Model file for the job. Use its own axes, mm. A direction names the side the tool comes from. Round coordinates to 2 decimals unless told otherwise and drop trailing zeros. Order: outer loops, then holes, each group sorted by start corner. A loop starts at its lowest first (then second) coordinate and runs counter-clockwise, first axis right, second up. Notation, with made-up numbers: (76, 41) - (80, 41) arc R27 cw to (80, 67) - close; hole circle Ø11 at (30.25, 72.5). An arc over 180 degrees is marked (long way). Answer as CSV lines item,"result". Start each with the question number.
1. Pin check, flat tips, straight feed: pin 1 Ø8 at (x, z) = (-31.5, 25.5) entering from -Y; pin 2 Ø6.5 at (x, y) = (2.5, 23.5) entering from +Z; pin 3 Ø15.5 at (x, y) = (5.5, -18) entering from +Z. Stop position of each tip, or through.
2. Band-saw the part on B-B on z = 22.5. List the corners of the cut face in (x, y).
3. Pull direction Y, two halves, no side cores. Call faces 3 (the face through (24.84, 19.39, 47.26)), 4 (the face through (-10, 22, 48)), 5 (the face through (43.14, -9.58, 25.32)), 6 (the face through (-37, 24, 0)): released by +Y, released by -Y, zero draft, split by the parting line, or undercut.
4. Band-saw the part on A-A on y = 0. List the corners of the cut face in (x, z).
5. Wall check: line 1 along X through (y, z) = (0, 47.4); line 2 along Z through (x, y) = (15.5, -3.5); line 3 along X through (y, z) = (22.5, 48.5). Give the ranges that are in metal, low to high. Write a range as [from, to].
6. 3-axis set-ups, long thin cutter, end or side, ignore diameter. For faces 1 (the face through (-1, 1, 2)), 2 (the face through (7.91, 12.21, 48.74)): which of +Z, -Z, +X, -X, +Y, -Y reach the whole face in a straight line?
```python
from build123d import *

# Parameters (mm, degrees)
F3_DEPTH = 1.5
F5_DEPTH = 1.5


with BuildPart() as f1:
    # F0 (on Right) → F1 (revolve)
    with BuildSketch(Plane.YZ):
        Polygon((0, 48), (0, 2), (42.57288, 2), (43.38192, 0), (45, 0), (44.19096, 2), (44.19096, 48), (45, 50), (43.38192, 50), (42.57288, 48), align=None)
    revolve(axis=Axis((0, 0, 25), (0, 0, 1)))

    # F2 (on face) → F3 (cut)
    with BuildSketch(Plane.XY.offset(48)):
        with BuildLine():
            ThreePointArc((-22.449944, 20), (-24.806967, 19.409586), (-26.607341, 17.777778))
            ThreePointArc((-26.607341, 17.777778), (0, -32), (26.607341, 17.777778))
            ThreePointArc((26.607341, 17.777778), (24.806967, 19.409586), (22.449944, 20))
            Line((22.449944, 20), (-22.449944, 20))
        make_face()
    extrude(amount=-F3_DEPTH, mode=Mode.SUBTRACT)

    # F4 (on face) → F5 (join)
    with BuildSketch(Plane.XY.offset(48)):
        with BuildLine():
            Line((1.90098, 39), (-1.90098, 39))
            ThreePointArc((-1.90098, 39), (-5.070925, 37.866711), (-6.803884, 34.980581))
            Line((-6.803884, 34.980581), (-9.846991, 19.765045))
            ThreePointArc((-9.846991, 19.765045), (-7.981844, 12.2941), (-1.021765, 9))
            Line((-1.021765, 9), (1.021765, 9))
            ThreePointArc((1.021765, 9), (7.981844, 12.2941), (9.846991, 19.765045))
            Line((9.846991, 19.765045), (6.803884, 34.980581))
            ThreePointArc((6.803884, 34.980581), (5.070925, 37.866711), (1.90098, 39))
        make_face()
        with BuildLine():
            ThreePointArc((7.88583, 19.372813), (6.43516, 13.562078), (1.021765, 11))
            Line((1.021765, 11), (-1.021765, 11))
            ThreePointArc((-1.021765, 11), (-6.43516, 13.562078), (-7.88583, 19.372813))
            Line((-7.88583, 19.372813), (-7.042723, 23.588348))
            ThreePointArc((-7.042723, 23.588348), (-6.002947, 25.320026), (-4.10098, 26))
            Line((-4.10098, 26), (4.10098, 26))
            ThreePointArc((4.10098, 26), (6.002947, 25.320026), (7.042723, 23.588348))
            Line((7.042723, 23.588348), (7.88583, 19.372813))
        make_face(mode=Mode.SUBTRACT)
    extrude(amount=F5_DEPTH)


solid = f1.part
```
Reply:
1,pin 1,"stops at y = -34.59"
1,pin 2,"stops at z = 49.5"
1,pin 3,"stops at z = 46.5"
2,outline,"circle Ø88.38 at (0, 0)"
3,face 3,"undercut"
3,face 4,"undercut"
3,face 5,"split by the parting line"
3,face 6,"zero draft"
4,outline,"(-45, 0) - (-43.38, 0) - (-42.57, 2) - (42.57, 2) - (43.38, 0) - (45, 0) - (44.19, 2) - (44.19, 48) - (45, 50) - (43.38, 50) - (42.57, 48) - (32, 48) - (32, 46.5) - (-32, 46.5) - (-32, 48) - (-42.57, 48) - (-43.38, 50) - (-45, 50) - (-44.19, 48) - (-44.19, 2) - close"
5,line 1,"x = [-44.19, -32], [32, 44.19]"
5,line 2,"z = [2, 46.5]"
5,line 3,"x = [-38.27, -36.38], [-9.3, -7.26], [7.26, 9.3], [36.38, 38.27]"
6,face 1,"-Z"
6,face 2,"+Z"
